Geometry: final body of the model. Coordinates: model frame, mm. Face numbers are marked on the shaded views. Give positions to 0.01 mm unless a question says otherwise; leave off trailing zeros. Order: outer loops, then holes, each group sorted by start corner. A loop starts at its lowest first (then second) coordinate and runs counter-clockwise, first axis right, second up. Notation, with made-up numbers: (81, 36.5) - (102, 36.5) arc R16 ccw to (102, 50.5) - close; hole circle Ø7 at (44, 33). An arc over 180 degrees is marked (long way). One line per item, written item: value.
```python
from build123d import *

# Parameters (mm, degrees)
F1_DEPTH = 2222
F2_R     = 7
F3_DEPTH = 75.001
F4_R     = 9
F5_DEPTH = 25


with BuildPart() as f1:
    # F0 (on Front) → F1 (new body)
    with BuildSketch(Plane.XZ):
        with BuildLine():
            Line((75, 0), (0, 0))
            Line((0, 0), (0, -12.5))
            Line((0, -12.5), (57, -12.5))
            ThreePointArc((57, -12.5), (65.485281, -16.014719), (69, -24.5))
            Line((69, -24.5), (69, -175.5))
            ThreePointArc((69, -175.5), (65.485281, -183.985281), (57, -187.5))
            Line((57, -187.5), (0, -187.5))
            Line((0, -187.5), (0, -200))
            Line((0, -200), (75, -200))
            Line((75, -200), (75, 0))
        make_face()
    extrude(amount=-F1_DEPTH)

    # F2 (on face) → F3 (cut, through all)
    with BuildSketch(Plane.YZ.offset(75)):
        Polygon((174, -200), (0, -83), (0, -200), align=None)
        Polygon((56, 0), (0, 0), (0, -83), align=None)
        Polygon((2222, -59), (2127, -200), (2222, -200), align=None)
        Polygon((2134, 0), (2222, -59), (2222, 0), align=None)
        with Locations((444, -75)):
            Circle(F2_R)
        with Locations((537, -138)):
            Circle(F2_R)
        with Locations((243, -138)):
            Circle(F2_R)
        with Locations((150, -75)):
            Circle(F2_R)
        with Locations((738, -75)):
            Circle(F2_R)
        with Locations((831, -138)):
            Circle(F2_R)
        with Locations((1032, -75)):
            Circle(F2_R)
        with Locations((1125, -138)):
            Circle(F2_R)
        with Locations((1326, -75)):
            Circle(F2_R)
        with Locations((1419, -138)):
            Circle(F2_R)
        with Locations((1620, -75)):
            Circle(F2_R)
        with Locations((1713, -138)):
            Circle(F2_R)
        with Locations((2007, -138)):
            Circle(F2_R)
        with Locations((1914, -75)):
            Circle(F2_R)
    extrude(amount=-F3_DEPTH, mode=Mode.SUBTRACT)

    # F4 (on face) → F5 (cut)
    with BuildSketch(Plane.XY):
        with Locations((37.5, 523)):
            Circle(F4_R)
        with Locations((37.5, 396)):
            Circle(F4_R)
        with Locations((37.5, 1757)):
            Circle(F4_R)
        with Locations((37.5, 1884)):
            Circle(F4_R)
    extrude(amount=-F5_DEPTH, mode=Mode.SUBTRACT)


solid = f1.part
```
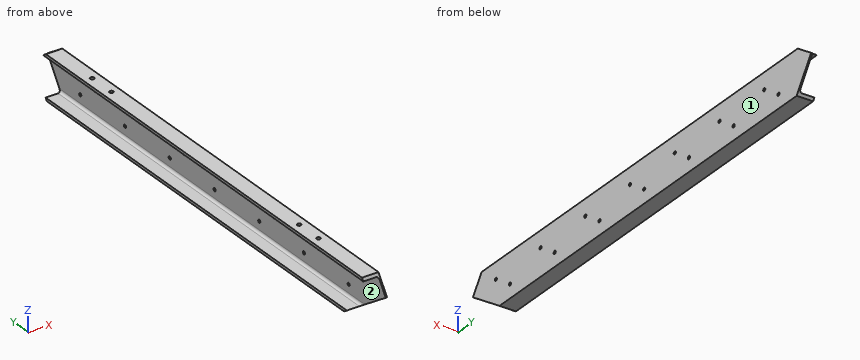
1) Material intervals for line 1 along Z through (x, y) = (48.5, 1633); line 2 along X through (y, z) = (1884, -2.5); line 3 along Z through (x, y) = (71.85, 2007), sorted ascending.
Answers below:
line 1: -200 to -187.5, -12.5 to 0
line 2: 0 to 28.5, 46.5 to 75
line 3: -200 to -145, -131 to 0
2) Mould query, pull axis Z, two halves, no side actions, for the marked faces 1 and 2. Classes: released by +Z, released by -Z, zero draft, split by the parting line, or undercut.
Answers below:
face 1: zero draft
face 2: undercut
3) Section B-B, the plane y = 1466.5. Return loops of the section in (x, z), then the cut area to 3 significant figures.
Answers below:
outline: (0, -200) - (75, -200) - (75, 0) - (0, 0) - (0, -12.5) - (57, -12.5) arc R12 cw to (69, -24.5) - (69, -175.5) arc R12 cw to (57, -187.5) - (0, -187.5) - close
area: 2,990 mm^2
4) Section A-A, the plane x = 12.5. Return loops of the section in (y, z).
Answers below:
outline: (47.57, -12.5) - (2152.64, -12.5) - (2134, 0) - (56, 0) - close; (155.41, -187.5) - (174, -200) - (2127, -200) - (2135.42, -187.5) - close
5) First-contact query: pin 1 (8 mm diameter, centred on y = 1536.5, z = -54.5, fed in from -X); pin 2 (11 mm diameter, centred on y = 831, z = -138, fed in from +X). Flat tips, straight axial feed; report the tip coordinate or a pass-through.
Answers below:
pin 1: x = 69
pin 2: through
